Geometry: see drawing. Coordinates: mm, zero at the bounding-box minimum. A direction names the side the tool comes from. Round coordinates to 2 decimals unless told otherwise and drop trailing zeros. Write each loop counter-clockwise with the first axis right and the second up, starting at its lowest first coordinate (ties: lowest second). Pieces come first, ordered by that corner, then holes. Notation, with made-up numbers: (16.25, 61.5) -> (75.25, 61.5) arc R26 cw to (75.25, 85.5) -> close; hole circle Ø10 at (-1, 13.25). An arc over 180 degrees is marked (long way). Use CSV: the item, a comma, the result in double quotes.
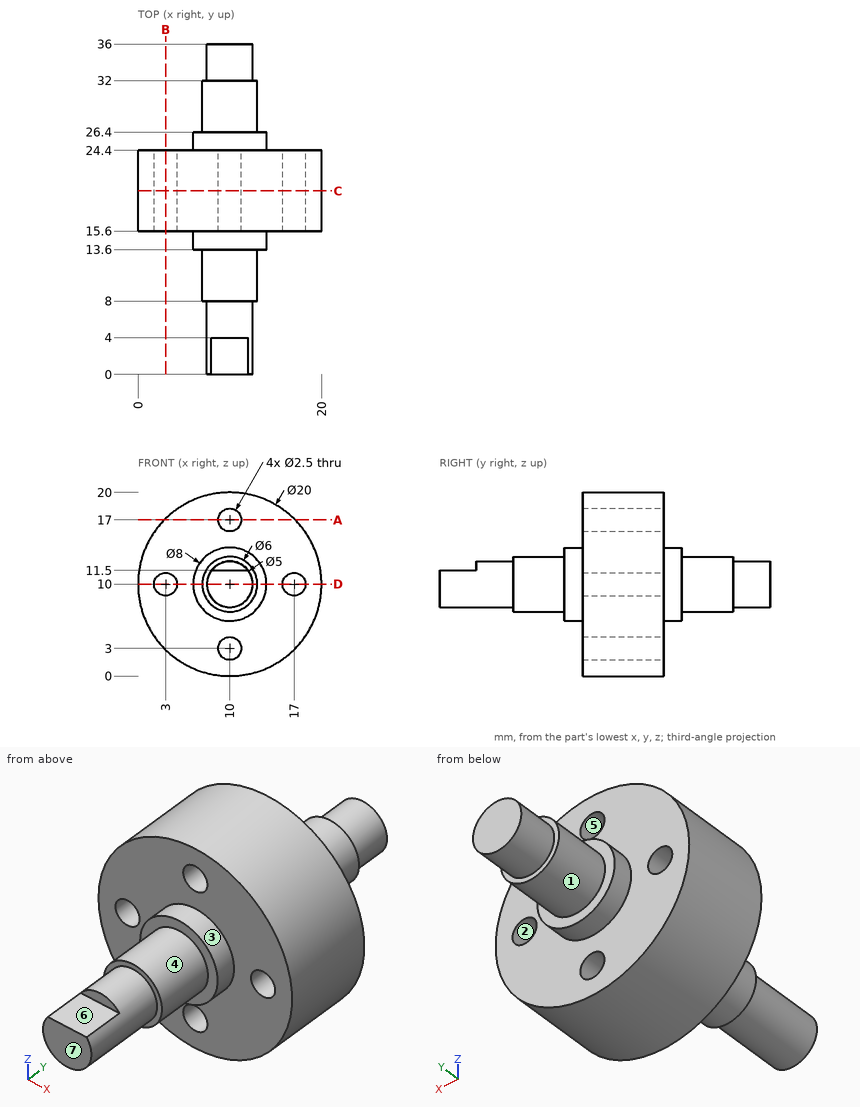
Item 1: Section query C-C on y = 20. Return the cut outline in (x, z), plus the area to 3 significant figures.
Worked answers:
outline,"circle Ø20 at (10, 10); hole circle Ø2.5 at (3, 10); hole circle Ø2.5 at (10, 3); hole circle Ø2.5 at (10, 17); hole circle Ø2.5 at (17, 10)"
area,"295 mm²"
Item 2: Section query B-B on x = 3. Return the cut outline in (y, z).
Worked answers:
outline,"(15.6, 2.86) -> (24.4, 2.86) -> (24.4, 8.75) -> (15.6, 8.75) -> close; (15.6, 11.25) -> (24.4, 11.25) -> (24.4, 17.14) -> (15.6, 17.14) -> close"
Item 3: Pull-direction query (Z, two-part tool) for the marked faces 4, 5, 6 and 7; classes: +Z half, -Z half, draft (parallel to the pull), parting line (faces both ways), or undercut.
Worked answers:
face 4,"parting line"
face 5,"undercut"
face 6,"+Z half"
face 7,"draft"
Item 4: First-contact query: pin 1 Ø8 at (x, y) = (13.5, 12) entering from +Z; pin 2 Ø5 at (y, z) = (9.5, 7.5) entering from +X; pin 3 Ø3 at (x, z) = (17, 10) entering from +Y; pin 4 Ø4 at (x, y) = (16.5, 7.5) entering from +Z. Flat tips, straight axial feed; report the tip coordinate or a pass-through.
Worked answers:
pin 1,"stops at z = 19.84"
pin 2,"stops at x = 13"
pin 3,"stops at y = 24.4"
pin 4,"passes through"
Item 5: Set-up query: the marked faces 1, 2 and 3. Return all of +Z, -Z, +X, -X, +Y, -Y with unobstructed straight access to the full face (end or side cutting, diameter ignored); none if empty.
Worked answers:
face 1,"+Y"
face 2,"+Y, -Y"
face 3,"-Y"
Item 6: Line query: line 1 (Y direction, x = 1.75, z = 5.25); line 2 (Z direction, x = 10, y = 3); line 3 (Y direction, x = 12.5, z = 12). Output: solid intervals per line, ascending.
Worked answers:
line 1,"y = 15.6 to 24.4"
line 2,"z = 7.5 to 11.5"
line 3,"y = 13.6 to 26.4"
Item 7: Section query D-D on z = 10. Give the number of separate pieces and of enclosed holes in the cut face, plus the area to 3 significant figures.
Worked answers:
separate pieces,"3"
enclosed holes,"0"
area,"291 mm²"
Item 8: Section query A-A on z = 17. Return the cut outline in (x, y), plus the area to 3 significant figures.
Worked answers:
outline,"(2.86, 15.6) -> (8.75, 15.6) -> (8.75, 24.4) -> (2.86, 24.4) -> close; (11.25, 15.6) -> (17.14, 15.6) -> (17.14, 24.4) -> (11.25, 24.4) -> close"
area,"104 mm²"
